```python
from build123d import *

# Parameters (mm, degrees)
BOX002_W       = 7
BOX002_H       = 1.6
BOX002_DEPTH   = 3
BOX001_W       = 7
BOX001_H       = 5
BOX001_DEPTH   = 1.7
BOX_W          = 10
BOX_H          = 7
BOX_DEPTH      = 10
CYLINDER_R     = 2.2
CYLINDER_DEPTH = 9


with BuildPart() as obj1:
    # Box002 → Box002 (new body)
    with BuildSketch(Plane(origin=(1, -2.6, -1.5), x_dir=(1, 0, 0), z_dir=(0, 0, 1))):
        with Locations((3.5, 0.8)):
            Rectangle(BOX002_W, BOX002_H)
    extrude(amount=BOX002_DEPTH)


with BuildPart() as obj2:
    # Box001 → Box001 (new body)
    with BuildSketch(Plane(origin=(1, -4, -0.85), x_dir=(1, 0, 0), z_dir=(0, 0, 1))):
        with Locations((3.5, 2.5)):
            Rectangle(BOX001_W, BOX001_H)
    extrude(amount=BOX001_DEPTH)


with BuildPart() as obj3:
    # Box → Box (new body)
    with BuildSketch(Plane(origin=(0, -0.5, -4), x_dir=(1, 0, 0), z_dir=(0, 0, 1))):
        with Locations((5, 3.5)):
            Rectangle(BOX_W, BOX_H)
    extrude(amount=BOX_DEPTH)


with BuildPart() as body:
    # Sketch → Revolution (revolve)
    with BuildSketch(Plane.XY):
        with BuildLine():
            add(Edge.make_bspline(
                [(1.699821, 2.2), (2.24, 1.1), (2.24, 0)],
                knots=[-2.2, -2.2, -2.2, 0, 0, 0], degree=2))
            Line((2.24, 0), (1.699821, 0))
            Line((1.699821, 0), (1.699821, 2.2))
        make_face()
    revolve(axis=Axis((0, 0, 0), (1, 0, 0)))


with BuildPart() as body_1:
    # Body placement: moved
    add(body.part.moved(Location((-1.7, 0, 0))))


with BuildPart() as cut003:
    # Cylinder → Cylinder (new body)
    with BuildSketch(Plane(origin=(0, 0, 0), x_dir=(0, 0, -1), z_dir=(1, 0, 0))):
        Circle(CYLINDER_R)
    extrude(amount=CYLINDER_DEPTH)

    # Cut: cut Body
    add(body_1.part, mode=Mode.SUBTRACT)

    # Cut001: cut obj3
    add(obj3.part, mode=Mode.SUBTRACT)

    # Cut002: cut obj2
    add(obj2.part, mode=Mode.SUBTRACT)

    # Cut003: cut obj1
    add(obj1.part, mode=Mode.SUBTRACT)


solid = cut003.part
```
Input: part model. Units: mm. Frame: model coordinates. A direction names the side the tool comes from. Round coordinates to 2 decimals unless told otherwise and drop trailing zeros. Loops run counter-clockwise (first coordinate to the right, second up) from the corner with the lowest first, then second, coordinate; pieces in that order, holes last. Notation, with made-up numbers: M -25.5,-28 L -11.5,-28 A20 ccw -11.5,-17 Z; hole C 16.5,70 d8. An arc over 180 degrees is marked long. Answer in a Markdown table with one row per item. Add a question column.
1. Set-up query: faces 4 (the face through (1, -1, 0)), 5 (the face through (9, -1, 0)). Return all of +Z, -Z, +X, -X, +Y, -Y with unobstructed straight access to the full face (end or side cutting, diameter ignored); none if empty.
2. Ray query, probe 1 along Z at (x, y) = (2.75, -1.1); probe 2 along X at (y, z) = (-1.55, 1.3); probe 3 along Z at (x, y) = (5.75, -1.4). Return the intervals inside material, ascending.
3. Section A-A (x = 4.75). Output: boundary loops of the cut face in (y, z).
4. Contact query for flat-ended pins moving along their axis: pin 1 (0.7 mm diameter, centred on x = 4.5, y = -1.5, fed in from -Z); pin 2 (0.8 mm diameter, centred on y = -1, z = 0, fed in from -X); pin 3 (0.7 mm diameter, centred on x = 4, y = -1, fed in from +Z). Output: stop coordinate, or through.
5. Mould query, pull axis Z, two halves, no side actions, for faces 1 (the face through (4.437, -1.345, 1.741)), 2 (the face through (8, -1, 0)), 3 (the face through (4, -0.5, 1)). Classes: released by +Z, released by -Z, zero draft, split by the parting line, or undercut.
Values follow:
| question | item | result |
|---|---|---|
| 1 | face 4 | -Y |
| 1 | face 5 | +Z, -Z, +X, +Y, -Y |
| 2 | probe 1 | -1.91 to -1.5, 1.5 to 1.91 |
| 2 | probe 2 | 0.08 to 1, 8 to 9 |
| 2 | probe 3 | -1.7 to -1.5, 1.5 to 1.7 |
| 3 | outline | M -1.61,-1.5 A2.2 ccw -0.5,-2.14 L -0.5,-0.85 L -1,-0.85 L -1,-1.5 Z; M -1.61,1.5 L -1,1.5 L -1,0.85 L -0.5,0.85 L -0.5,2.14 A2.2 ccw Z |
| 4 | pin 1 | z = -1.88 |
| 4 | pin 2 | x = 0.32 |
| 4 | pin 3 | z = 2.1 |
| 5 | face 1 | split by the parting line |
| 5 | face 2 | undercut |
| 5 | face 3 | zero draft |
